```python
from build123d import *

# Parameters (mm, degrees)
SKETCH_1_R        = 2
EXTRUDE_2_DEPTH   = 8.5
SKETCH_1_R_2      = 3.9
EXTRUDE_2_2_DEPTH = 8.5
SKETCH_1_6_R      = 1.5
SKETCH_1_6_R_2    = 3.9
EXTRUDE_3_DEPTH   = 1.8
SKETCH_1_7_R      = 1.5
EXTRUDE_4_DEPTH   = 13.8


with BuildPart() as part:
    # Sketch 1 → Extrude 2 (new body)
    with BuildSketch(Plane(origin=(0, 0, 0), x_dir=(0, 0, -1), z_dir=(1, 0, 0))):
        Polygon((-6.85, 38.325), (-6.85, 22.325), (-29.85, 22.325), (-29.85, -22.325), (-6.85, -22.325), (-6.85, -38.325), (19.061824645, -38.325), (26.35, -36.675), (28.35, -36.675), (28.35, -17.675), (29.85, -17.675), (29.85, 17.325), (35.35, 17.325), (35.35, 36.325), (26.35, 36.325), (19.15, 38.325), align=None)
        with Locations((-25.9, -18.375)):
            Circle(SKETCH_1_R, mode=Mode.SUBTRACT)
        with BuildLine():
            Line((-5.05, -36.525), (-5.05, -20.525))
            Line((-5.05, -20.525), (-21.085438753, -20.525))
            ThreePointArc((-21.085438753, -20.525), (-21.87039838, -20.144546918), (-22.058077389, -19.292676768))
            ThreePointArc((-22.058077389, -19.292676768), (-22.783982594, -15.947463074), (-25.85, -14.425316468))
            Line((-25.85, -14.425316468), (-25.85, 2.325))
            Line((-25.85, 2.325), (-28.05, 2.325))
            Line((-28.05, 2.325), (-28.05, 13.560438753))
            ThreePointArc((-28.05, 13.560438753), (-27.669546918, 14.34539838), (-26.817676768, 14.533077389))
            ThreePointArc((-26.817676768, 14.533077389), (-23.106928214, 15.581928214), (-22.058077389, 19.292676768))
            ThreePointArc((-22.058077389, 19.292676768), (-21.87039838, 20.144546918), (-21.085438753, 20.525))
            Line((-21.085438753, 20.525), (-5.05, 20.525))
            Line((-5.05, 20.525), (-5.05, 36.125))
            Line((-5.05, 36.125), (19.15, 36.125))
            Line((19.15, 36.125), (26.35, 34.525))
            Line((26.35, 34.525), (33.55, 34.525))
            Line((33.55, 34.525), (33.55, 19.125))
            Line((33.55, 19.125), (28.05, 19.125))
            Line((28.05, 19.125), (28.05, -15.875))
            Line((28.05, -15.875), (26.268653348, -15.875))
            ThreePointArc((26.268653348, -15.875), (20.582582899, -18.821924489), (25.325510204, -23.125458115))
            ThreePointArc((25.325510204, -23.125458115), (26.172699849, -23.317473758), (26.55, -24.099934555))
            Line((26.55, -24.099934555), (26.55, -34.875))
            Line((26.55, -34.875), (19.061824645, -36.525))
            Line((19.061824645, -36.525), (-5.05, -36.525))
        make_face(mode=Mode.SUBTRACT)
        with Locations((24.45, -19.325)):
            Circle(SKETCH_1_R, mode=Mode.SUBTRACT)
        with Locations((-25.9, 18.375)):
            Circle(SKETCH_1_R, mode=Mode.SUBTRACT)
    extrude(amount=EXTRUDE_2_DEPTH)



with BuildPart() as body_2:
    # Sketch 1 → Extrude 2 2 (new body)
    with BuildSketch(Plane(origin=(0, 0, 0), x_dir=(0, 0, -1), z_dir=(1, 0, 0))):
        with Locations((25.35, 28.825)):
            Circle(SKETCH_1_R_2)
        with Locations((25.35, 28.825)):
            Circle(SKETCH_1_R, mode=Mode.SUBTRACT)
    extrude(amount=EXTRUDE_2_2_DEPTH)


with BuildPart() as part_1:
    add(part.part)

    add(body_2.part)  # Extrude 3 merges body 2
    # Sketch 1_6 → Extrude 3 (add)
    with BuildSketch(Plane(origin=(0, 0, 0), x_dir=(0, 0, -1), z_dir=(1, 0, 0))):
        with BuildLine():
            Line((-21.085438753, -20.525), (-5.05, -20.525))
            Line((-5.05, -20.525), (-5.05, -36.525))
            Line((-5.05, -36.525), (19.061824645, -36.525))
            Line((19.061824645, -36.525), (26.55, -34.875))
            Line((26.55, -34.875), (26.55, -24.099934555))
            ThreePointArc((26.55, -24.099934555), (26.172699849, -23.317473758), (25.325510204, -23.125458115))
            ThreePointArc((25.325510204, -23.125458115), (20.582582899, -18.821924489), (26.268653348, -15.875))
            Line((26.268653348, -15.875), (26.55, -15.875))
            Line((26.55, -15.875), (28.05, -15.875))
            Line((28.05, -15.875), (28.05, 19.125))
            Line((28.05, 19.125), (33.55, 19.125))
            Line((33.55, 19.125), (33.55, 34.525))
            Line((33.55, 34.525), (26.35, 34.525))
            Line((26.35, 34.525), (19.15, 36.125))
            Line((19.15, 36.125), (-5.05, 36.125))
            Line((-5.05, 36.125), (-5.05, 20.525))
            Line((-5.05, 20.525), (-21.085438753, 20.525))
            ThreePointArc((-21.085438753, 20.525), (-21.87039838, 20.144546918), (-22.058077389, 19.292676768))
            ThreePointArc((-22.058077389, 19.292676768), (-23.106928214, 15.581928214), (-26.817676768, 14.533077389))
            ThreePointArc((-26.817676768, 14.533077389), (-27.669546918, 14.34539838), (-28.05, 13.560438753))
            Line((-28.05, 13.560438753), (-28.05, 2.325))
            Line((-28.05, 2.325), (-25.85, 2.325))
            Line((-25.85, 2.325), (-25.85, -14.425316468))
            ThreePointArc((-25.85, -14.425316468), (-22.783982594, -15.947463074), (-22.058077389, -19.292676768))
            ThreePointArc((-22.058077389, -19.292676768), (-21.87039838, -20.144546918), (-21.085438753, -20.525))
        make_face()
        with Locations((-0.85, -16.475)):
            Circle(SKETCH_1_6_R, mode=Mode.SUBTRACT)
        with Locations((-2.55, 18.525)):
            Circle(SKETCH_1_6_R, mode=Mode.SUBTRACT)
        with Locations((25.35, 28.825)):
            Circle(SKETCH_1_6_R_2, mode=Mode.SUBTRACT)
    extrude(amount=EXTRUDE_3_DEPTH)

    # Sketch 1_7 → Extrude 4 (add)
    with BuildSketch(Plane(origin=(0, 0, 0), x_dir=(0, 0, -1), z_dir=(1, 0, 0))):
        with Locations(Location((-2.55, 18.525, 0), (0, 0, 180))):
            Circle(SKETCH_1_7_R)
        with Locations(Location((-0.85, -16.475, 0), (0, 0, 180))):
            Circle(SKETCH_1_7_R)
    extrude(amount=EXTRUDE_4_DEPTH)


solid = part_1.part
```
Geometry: final body of the model. Coordinates: model frame, mm. A direction names the side the tool comes from. Round coordinates to 2 decimals unless told otherwise and drop trailing zeros. Write each loop counter-clockwise with the first axis right and the second up, starting at its lowest first coordinate (ties: lowest second). Pieces come first, ordered by that corner, then holes. Notation, with made-up numbers: (-25, -2.5) -> (12, -2.5) arc R30 cw to (12, 24.5) -> close; hole circle Ø11 at (66, 77). An arc over 180 degrees is marked (long way). Use CSV: the item, a comma, the result in double quotes. Start each with the question number.
Q1. Section A-A (z = -24.45). Return loops of the section in (x, y) (3 decimals).
Q2. Reachability of faces 1 (the face through (7.72, -17.96, 0.65)), 2 (the face through (4, 36.325, -31)), 3 (the face through (4, 30, 6.85)), 4 (the face through (4, -30, 6.85)), 5 (the face through (4, -36.675, -27)) from +Z, -Z, +X, -X, +Y, -Y: full face, straight path, thin tool, end or side. Return the list, or none.
Q3. Line query: L1, parallel to Y at x = 6, z = 25.9 (3 decimals); L2, parallel to Z at x = 7.75, y = 13; L3, parallel to Y at x = 7.5, z = 18 (3 decimals). Output: solid intervals per line, ascending.
Q4. Section D-D (x = 10.75). Return loops of the section in (y, z) (3 decimals), plus the area to 3 significant figures.
Q5. Section C-C (z = -17). Return loops of the section in (x, y) (3 decimals).
Q6. Pull-direction query (Z, two-part tool) for faces 6 (the face through (5.1, 15.54, 23.15)), 7 (the face through (5, -36.525, -7)), 8 (the face through (0, 1, -2)), 9 (the face through (4, 0, -29.85)); classes: pulls with the +Z half, pulls with the -Z half, needs draft (parallel to the pull), parting line crosses it, or undercut.
Q7. Section B-B (y = -1). Return loops of the section in (x, z), plus the area to 3 significant figures.
Q8. First-contact query: pin 1 Ø7 at (x, y) = (3.5, -23.5) entering from -Z; pin 2 Ø5.5 at (x, y) = (6.5, 9) entering from -Z; pin 3 Ø4.5 at (x, z) = (5, -32) entering from +Y (3 decimals); pin 4 Ø3 at (y, z) = (-24.5, 9.5) entering from -X. Flat tips, straight axial feed; report the tip coordinate or a pass-through.
Result sheet:
1,outline,"(0, -37.105) -> (8.5, -37.105) -> (8.5, -35.338) -> (1.8, -35.338) -> (1.8, -23.225) -> (8.5, -23.225) -> (8.5, -21.325) -> (0, -21.325) -> close; (0, -17.325) -> (8.5, -17.325) -> (8.5, -15.425) -> (1.8, -15.425) -> (1.8, 25.03) -> (8.5, 25.03) -> (8.5, 27.039) -> (0, 27.039) -> close; (0, 30.611) -> (8.5, 30.611) -> (8.5, 32.62) -> (1.8, 32.62) -> (1.8, 34.947) -> (8.5, 34.947) -> (8.5, 36.853) -> (0, 36.853) -> close"
2,face 1,"+X"
2,face 2,"-Z, +X, -X, +Y"
2,face 3,"+Z, +X, -X, +Y"
2,face 4,"+Z, +X, -X, -Y"
2,face 5,"-Z, +X, -X, -Y"
3,L1,"-22.325 to -20.375, -16.375 to 2.325, 14.425 to 16.375, 20.375 to 22.325"
3,L2,"-29.85 to -28.05, 28.05 to 29.85"
3,L3,"-22.325 to -20.525, 20.525 to 22.325"
4,outline,"circle Ø3 at (-16.475, 0.85); circle Ø3 at (18.525, 2.55)"
4,area,"14.1 mm²"
5,outline,"(0, -38.325) -> (8.5, -38.325) -> (8.5, -36.525) -> (1.8, -36.525) -> (1.8, 36.125) -> (8.5, 36.125) -> (8.5, 38.325) -> (0, 38.325) -> close"
6,face 6,"undercut"
6,face 7,"undercut"
6,face 8,"needs draft"
6,face 9,"pulls with the -Z half"
7,outline,"(0, -29.85) -> (8.5, -29.85) -> (8.5, -28.05) -> (1.8, -28.05) -> (1.8, 25.85) -> (8.5, 25.85) -> (8.5, 29.85) -> (0, 29.85) -> close"
7,area,"146 mm²"
8,pin 1,"z = -28.35"
8,pin 2,"z = -29.85"
8,pin 3,"y = 36.325"
8,pin 4,"through"
